from build123d import *

# Parameters (mm, degrees)
SKETCH2_R           = 1.25
BOSS_EXTRUDE1_DEPTH = 2
BOSS_EXTRUDE2_DEPTH = 1
SKETCH3_R           = 0.15
CUT_EXTRUDE1_DEPTH  = 0.5


with BuildPart() as part:
    # Sketch2 → Boss-Extrude1 (new body)
    with BuildSketch(Plane.YZ):
        with BuildLine():
            ThreePointArc((-4.35, -14.45), (-3.075914484, -17.525914513), (4.1e-08, -18.8))
            ThreePointArc((4.1e-08, -18.8), (3.075914513, -17.525914484), (4.35, -14.45))
            Line((4.35, -14.45), (6.1, 0))
            Line((6.1, 0), (6.1, 0.55))
            ThreePointArc((6.1, 0.55), (6.070921356, 1.144906627), (5.983962658, 1.734141424))
            Line((5.983962658, 1.734141424), (3.25, 15.55))
            ThreePointArc((3.25, 15.55), (2.298097039, 17.848097039), (0, 18.8))
            ThreePointArc((0, 18.8), (-2.298097039, 17.848097039), (-3.25, 15.55))
            Line((-3.25, 15.55), (-5.983962658, 1.734141424))
            ThreePointArc((-5.983962658, 1.734141424), (-6.070921356, 1.144906627), (-6.1, 0.55))
            Line((-6.1, 0.55), (-6.1, 0))
            Line((-6.1, 0), (-4.35, -14.45))
        make_face()
        with BuildLine():
            Line((3.550344828, -0.045862069), (2.35, -14.45))
            ThreePointArc((2.35, -14.45), (0, -16.8), (-2.35, -14.45))
            Line((-2.35, -14.45), (-3.550344828, -0.045862069))
            ThreePointArc((-3.550344828, -0.045862069), (-3.58756473, 0.251036273), (-3.6, 0.55))
            ThreePointArc((-3.6, 0.55), (0, 4.15), (3.6, 0.55))
            ThreePointArc((3.6, 0.55), (3.58756473, 0.251036273), (3.550344828, -0.045862069))
        make_face(mode=Mode.SUBTRACT)
        with Locations(Location((0, 15.55, 0), (0, 0, 270))):
            Circle(SKETCH2_R, mode=Mode.SUBTRACT)
    extrude(amount=BOSS_EXTRUDE1_DEPTH)

    # Sketch2_3 → Boss-Extrude2 (add)
    with BuildSketch(Plane.YZ):
        with BuildLine():
            ThreePointArc((-2.35, -14.45), (0, -16.8), (2.35, -14.45))
            Line((2.35, -14.45), (3.550344828, -0.045862069))
            Line((3.550344828, -0.045862069), (3.6, 0.55))
            ThreePointArc((3.6, 0.55), (0, 4.15), (-3.6, 0.55))
            Line((-3.6, 0.55), (-3.550344828, -0.045862069))
            Line((-3.550344828, -0.045862069), (-2.35, -14.45))
        make_face()
    extrude(amount=BOSS_EXTRUDE2_DEPTH)

    # Sketch3 → Cut-Extrude1 (cut)
    with BuildSketch(Plane.YZ.offset(1)):
        with Locations(Location((0, 0.55, 0), (0, 0, 270))):
            Circle(SKETCH3_R)
        with Locations(Location((0, -14.45, 0), (0, 0, 270))):
            Circle(SKETCH3_R)
    extrude(amount=-CUT_EXTRUDE1_DEPTH, mode=Mode.SUBTRACT)


solid = part.part
Geometry: final body of the model. Coordinates: model frame, mm. A direction names the side the tool comes from. Give positions to 0.01 mm unless a question says otherwise; leave off trailing zeros. Order: outer loops, then holes, each group sorted by start corner. A loop starts at its lowest first (then second) coordinate and runs counter-clockwise, first axis right, second up. Notation, with made-up numbers: (-27, -30) -> (-11, -30) arc R34 cw to (-11, 8) -> close; hole circle Ø4 at (70.25, -14.75). An arc over 180 degrees is marked (long way). Write each question's results on one line, items separated by ' | '.
1) Cut plane B-B (z = -15). Output: boundary loops of the cut face in (x, y).
Geometry says:
outline: (0, -4.32) -> (2, -4.32) -> (2, -2.28) -> (1, -2.28) -> (1, 2.28) -> (2, 2.28) -> (2, 4.32) -> (0, 4.32) -> close
2) Cut plane A-A (x = 1.35). Output: boundary loops of the cut face in (y, z).
Geometry says:
outline: (-6.1, 0) -> (-4.35, -14.45) arc R4.35 ccw to (4.35, -14.45) -> (6.1, 0) -> (6.1, 0.55) arc R6.1 ccw to (5.98, 1.73) -> (3.25, 15.55) arc R3.25 ccw to (-3.25, 15.55) -> (-5.98, 1.73) arc R6.1 ccw to (-6.1, 0.55) -> close; hole (-3.55, -0.05) -> (-2.35, -14.45) arc R2.35 ccw to (2.35, -14.45) -> (3.55, -0.05) arc R3.6 ccw (long way) to start; hole circle Ø2.5 at (0, 15.55)
3) Cut plane D-D (z = -11). Output: boundary loops of the cut face in (x, y), and give its area (3 significant figures).
Geometry says:
outline: (0, -4.77) -> (2, -4.77) -> (2, -2.64) -> (1, -2.64) -> (1, 2.64) -> (2, 2.64) -> (2, 4.77) -> (0, 4.77) -> close | area: 13.8 mm²
4) Draft query along Y for faces 1 (the face through (1.49, -2.94, -7.35)), 2 (the face through (2, -0.1, 4.4)), 3 (the face through (0.986, -4.598, 8.739)). Return one class per face: released by +Y, released by -Y, zero draft, split by the parting line, or undercut.
Geometry says:
face 1: undercut | face 2: zero draft | face 3: released by -Y
5) Cut plane C-C (y = -5). Output: boundary loops of the cut face in (x, z), and give its area (3 significant figures).
Geometry says:
outline: (0, -9.08) -> (2, -9.08) -> (2, 6.71) -> (0, 6.71) -> close | area: 31.6 mm²
6) Line query: line 1 along Y through (x, z) = (0.7, -14.45); line 2 along Z through (x, y) = (1.45, -0.75); line 3 along Z through (x, y) = (1.2, 1). Output: solid intervals per line, ascending.
Geometry says:
line 1: y = -4.35 to -0.15, 0.15 to 4.35 | line 2: z = -18.73 to -16.68, 4.07 to 14.55, 16.55 to 18.71 | line 3: z = -18.68 to -16.58, 4.01 to 14.8, 16.3 to 18.64
7) First-contact query: pin 1 Ø2 at (y, z) = (0, 15.55) entering from +X; pin 2 Ø6 at (y, z) = (-0.5, -7) entering from -X; pin 3 Ø1 at (x, y) = (0.5, 3) entering from +Z; pin 4 Ø3.5 at (y, z) = (0.5, -8) entering from +X. Flat tips, straight axial feed; report the tip coordinate or a pass-through.
Geometry says:
pin 1: passes through | pin 2: stops at x = 0 | pin 3: stops at z = 17.63 | pin 4: stops at x = 1
8) Set-up query: faces 4 (the face through (0.986, 5.213, -7.326)), 5 (the face through (1.49, 2.96, -7.15)). Return all of +Z, -Z, +X, -X, +Y, -Y with unobstructed straight access to the full face (end or side cutting, diameter ignored); none if empty.
Geometry says:
face 4: -Z, +X, -X, +Y | face 5: +X
